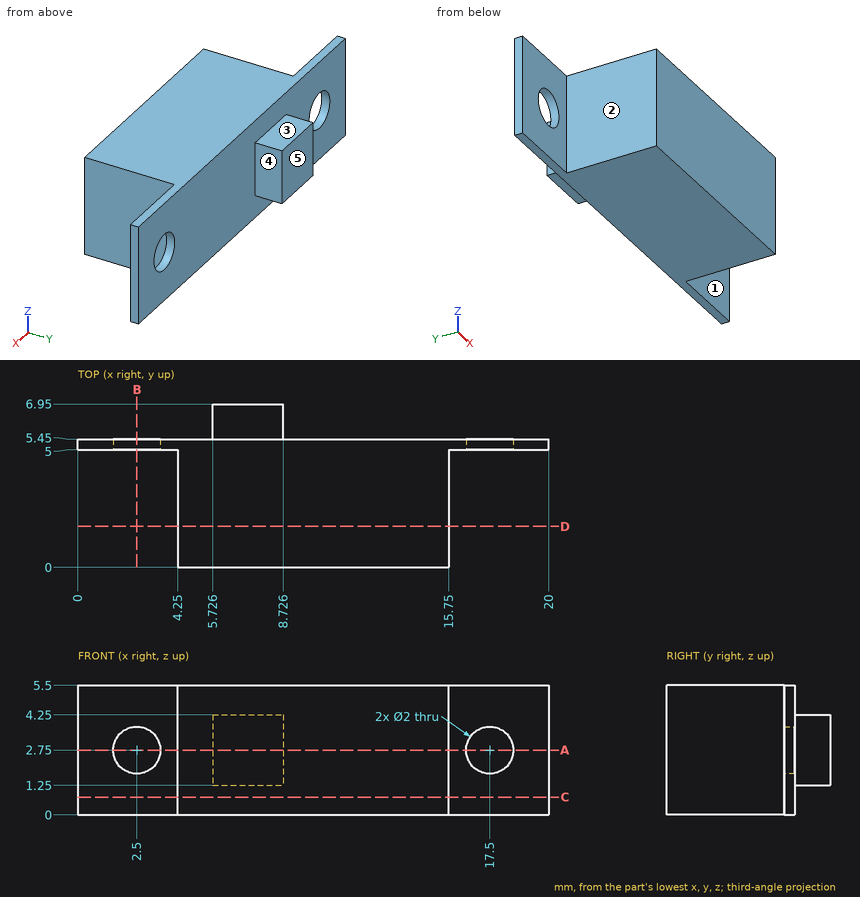
The drawing under review shows one solid part. Ordinate dimensions are in mm from its lowest x, y, z. A direction names the side the tool comes from. Round coordinates to 2 decimals unless told otherwise and drop trailing zeros. Write each loop counter-clockwise with the first axis right and the second up, starting at its lowest first coordinate (ties: lowest second). Pieces come first, ordered by that corner, then holes. Notation, with made-up numbers: (34, 83) - (87, 83) arc R9 ccw to (87, 94) - close; hole circle Ø5 at (70.5, -11). An arc over 180 degrees is marked (long way). Use a Markdown table: item, result. Add a question column.
1. For the marked faces 1, 2, 3, 4 and 5, list the 3-axis set-ups (+Z, -Z, +X, -X, +Y, -Y) from which the entire face can be reached by the end or side of a thin tool; tool diameter is ignored.
2. We need section C-C (z = 0.75). State the section outline as (x, y) points.
3. We need section A-A (z = 2.75). State the section outline as (x, y) points, then the cut area to 3 significant figures.
4. Wall thickness on probe 1 along X at (y, z) = (5.4, 2.75); probe 2 along X at (y, z) = (2.5, 2.9); probe 3 along Y at (x, z) = (11.25, 2.8): over which ranges is each line inside the solid? List them lowest first.
5. Clearance check with flat-ended pins moving along their axes: pin 1 (2.5 mm diameter, centred on y = 3.5, z = 1.5, fed in from -X); pin 2 (3 mm diameter, centred on x = 13.5, z = 2, fed in from +Y); pin 3 (2 mm diameter, centred on x = 2.5, z = 3.5, fed in from -Y); pin 4 (1.8 mm diameter, centred on x = 2.5, z = 2.75, fed in from -Y). State where each tip first meets the part, or that it passes through.
6. We need section D-D (y = 1.75). State the section outline as (x, z) points.
7. We need section B-B (x = 2.5). State the section outline as (y, z) points.
Output:
| question | item | result |
|---|---|---|
| 1 | face 1 | +Z, -Z, +X, -Y |
| 1 | face 2 | +Z, -Z, -X, -Y |
| 1 | face 3 | +Z, +X, -X, +Y |
| 1 | face 4 | +Z, -Z, +X, +Y |
| 1 | face 5 | +Z, -Z, +X, -X, +Y |
| 2 | outline | (0, 5) - (4.25, 5) - (4.25, 0) - (15.75, 0) - (15.75, 5) - (20, 5) - (20, 5.45) - (0, 5.45) - close |
| 3 | outline | (0, 5) - (1.5, 5) - (1.5, 5.45) - (0, 5.45) - close; (3.5, 5) - (4.25, 5) - (4.25, 0) - (15.75, 0) - (15.75, 5) - (16.5, 5) - (16.5, 5.45) - (8.73, 5.45) - (8.73, 6.95) - (5.73, 6.95) - (5.73, 5.45) - (3.5, 5.45) - close; (18.5, 5) - (20, 5) - (20, 5.45) - (18.5, 5.45) - close |
| 3 | area | 69.2 mm2 |
| 4 | probe 1 | x = 0 to 1.5, 3.5 to 16.5, 18.5 to 20 |
| 4 | probe 2 | x = 4.25 to 15.75 |
| 4 | probe 3 | y = 0 to 5.45 |
| 5 | pin 1 | stops at x = 4.25 |
| 5 | pin 2 | stops at y = 5.45 |
| 5 | pin 3 | stops at y = 5 |
| 5 | pin 4 | passes through |
| 6 | outline | (4.25, 0) - (15.75, 0) - (15.75, 5.5) - (4.25, 5.5) - close |
| 7 | outline | (5, 0) - (5.45, 0) - (5.45, 1.75) - (5, 1.75) - close; (5, 3.75) - (5.45, 3.75) - (5.45, 5.5) - (5, 5.5) - close |
